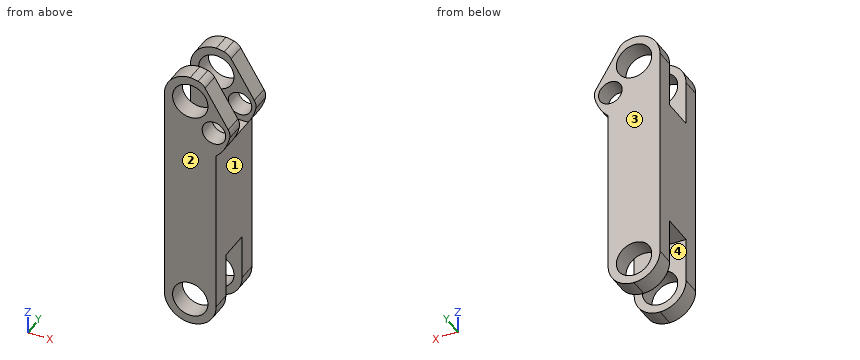
from build123d import *

# Parameters (mm, degrees)
F1_DEPTH = 147
F2_R     = 37.5
F2_R_2   = 25
F3_DEPTH = 147.001
F5_DEPTH = 147.001
F6_R     = 25
F7_W     = 67.6
F7_H     = 95
F7_H_2   = 55
F8_DEPTH = 139.2839551991


with BuildPart() as f1:
    # F0 (on Front) → F1 (new body)
    with BuildSketch(Plane.XZ):
        with BuildLine():
            Line((55, -229.4613795656), (55, 120.3808841783))
            ThreePointArc((55, 120.3808841783), (80.7033356829, 220.2549606622), (0, 284.4613795656))
            ThreePointArc((0, 284.4613795656), (-38.8908729653, 268.3522525309), (-55, 229.4613795656))
            Line((-55, 229.4613795656), (-55, -229.4613795656))
            ThreePointArc((-55, -229.4613795656), (-38.8908729653, -268.3522525309), (0, -284.4613795656))
            ThreePointArc((0, -284.4613795656), (38.8908729653, -268.3522525309), (55, -229.4613795656))
        make_face()
    extrude(amount=F1_DEPTH)

    # F2 (on face) → F3 (cut, through all)
    with BuildSketch(Plane.XZ.offset(147)):
        with Locations((0, 229.4613795656)):
            Circle(F2_R)
        with Locations((0, -229.4613795656)):
            Circle(F2_R)
        with Locations((50.271846354, 172.1997708082)):
            Circle(F2_R_2)
    extrude(amount=-F3_DEPTH, mode=Mode.SUBTRACT)

    # F4 (on face) → F5 (cut, through all)
    with BuildSketch(Plane.XZ.offset(147)):
        with BuildLine():
            ThreePointArc((85.2657948536, 181.983535776), (71.7102726141, 239.5566412204), (26.6566362615, 277.878756312))
            Line((26.6566362615, 277.878756312), (85.2657948536, 181.983535776))
        make_face()
    extrude(amount=-F5_DEPTH, mode=Mode.SUBTRACT)

    # F6
    f6_edges = [f1.edges().sort_by_distance(p)[0] for p in [
        (85.265795, -73.5, 181.983536),
        (26.656636, -73.5, 277.878756),
    ]]
    fillet(f6_edges, radius=F6_R)

    # F7 (on face) → F8 (cut, through all)
    with BuildSketch(Plane(origin=(-55, 0, 0), x_dir=(0, -1, 0), z_dir=(-1, 0, 0))):
        with Locations((73.5, -181.9613795656)):
            Rectangle(F7_W, F7_H)
        with Locations((73.5, -256.9613795656)):
            Rectangle(F7_W, F7_H_2)
        with Locations((73.5, 181.9613795656)):
            Rectangle(F7_W, F7_H)
        with Locations((73.5, 256.9613795656)):
            Rectangle(F7_W, F7_H_2)
    extrude(amount=-F8_DEPTH, mode=Mode.SUBTRACT)


solid = f1.part
Geometry check sheet. Reference: the model listing, model coordinates, mm. Face numbers are marked on the shaded views. Give positions to 0.01 mm unless a question says otherwise; leave off trailing zeros. Write each loop counter-clockwise with the first axis right and the second up, starting at its lowest first coordinate (ties: lowest second). Pieces come first, ordered by that corner, then holes. Notation, with made-up numbers: (36.25, 68.5) - (72.25, 68.5) arc R18 ccw to (72.25, 91.5) - close; hole circle Ø6 at (64, 81). An arc over 180 degrees is marked (long way). Put each result on its own line as item: value.
1. Sectioned sample at D-D, the plane z = 0. Enter the section's corners in (x, y), plus the area to 3 significant figures.
Ans:
outline: (-55, -147) - (55, -147) - (55, 0) - (-55, 0) - close
area: 16,200 mm²
2. Sectioned sample at C-C, the plane y = -26. Enter the section's corners in (x, z).
Ans:
outline: (-55, -229.46) arc R55 ccw to (55, -229.46) - (55, 120.38) arc R94.77 ccw to (83.8, 171.69) arc R25 ccw to (80.61, 189.59) - (31.31, 270.27) arc R25 ccw to (16.83, 281.27) arc R94.77 ccw to (0, 284.46) arc R55 ccw to (-55, 229.46) - close; hole circle Ø75 at (0, -229.46); hole circle Ø75 at (0, 229.46); hole circle Ø50 at (50.27, 172.2)
3. Sectioned sample at A-A, the plane z = 159.5. Enter the section's corners in (x, y).
Ans:
outline: (-55, -147) - (28.74, -147) - (28.74, -107.3) - (-55, -107.3) - close; (-55, -39.7) - (28.74, -39.7) - (28.74, 0) - (-55, 0) - close; (71.81, -147) - (80.53, -147) - (80.53, -107.3) - (71.81, -107.3) - close; (71.81, -39.7) - (80.53, -39.7) - (80.53, 0) - (71.81, 0) - close
4. Sectioned sample at B-B, the plane y = -91. Enter the section's corners in (x, z), plus the area to 3 significant figures.
Ans:
outline: (-55, -134.46) - (55, -134.46) - (55, 120.38) arc R94.77 ccw to (67.54, 134.46) - (-55, 134.46) - close
area: 29,700 mm²
5. Go/stop test with flat-tipped pins: pin 1 (10 mm diameter, centred on x = 50.5, y = -111, fed in from +Z); pin 2 (12 mm diameter, centred on y = -103, z = -107.5, fed in from +X); pin 3 (12 mm diameter, centred on x = 64.5, y = -119.5, fed in from -Z). Record where each tip stops, or that it passes through.
Ans:
pin 1: stops at z = 247.05
pin 2: stops at x = 55
pin 3: stops at z = 123.77
6. Thickness scan on line 1 (Z direction, x = 0, y = -125); line 2 (Z direction, x = 0.5, y = -121.5); line 3 (Y direction, x = 34, z = -209). Record the ranges inside material, lowest first.
Ans:
line 1: z = -284.46 to -266.96, -191.96 to 191.96, 266.96 to 284.46
line 2: z = -284.46 to -266.96, -191.96 to 191.96, 266.96 to 284.41
line 3: y = -147 to -107.3, -39.7 to 0
7. Draft check along Y on the marked faces 1, 2, 3 and 4. Enter one of: +Y half, -Y half, draft (parallel to the pull), parting line (faces both ways), or undercut.
Ans:
face 1: draft
face 2: -Y half
face 3: +Y half
face 4: undercut
